```python
from build123d import *

# Parameters (mm, degrees)
F0_W     = 19.05
F0_H     = 3.429
F2_W     = 17.526
F2_H     = 2.413
F4_W     = 16.002
F4_H     = 2.413
F6_R     = 1.7399
F7_DEPTH = 8.256


with BuildPart() as f1:
    # F0 (on Front) → F1 (revolve)
    with BuildSketch(Plane.XZ):
        with Locations((9.525, 1.7145)):
            Rectangle(F0_W, F0_H)
    revolve(axis=Axis((0, 0, 1.7145), (0, 0, 1)))

    # F2 (on Front) → F3 (revolve)
    with BuildSketch(Plane.XZ):
        with Locations((8.763, 4.6355)):
            Rectangle(F2_W, F2_H)
    revolve(axis=Axis((0, 0, 4.6355), (0, 0, 1)))

    # F4 (on Front) → F5 (revolve)
    with BuildSketch(Plane.XZ):
        with Locations((8.001, 7.0485)):
            Rectangle(F4_W, F4_H)
    revolve(axis=Axis((0, 0, 7.0485), (0, 0, 1)))

    # F6 (on face) → F7 (cut, through all)
    with BuildSketch(Plane.XY.offset(8.255)):
        with Locations((8.243714, 4.308599)):
            Circle(F6_R)
    extrude(amount=-F7_DEPTH, mode=Mode.SUBTRACT)


solid = f1.part
```
Can you work these out from the model? Positions are in its coordinate system, mm. A direction names the side the tool comes from. Give positions to 0.01 mm unless a question says otherwise; leave off trailing zeros. Loops run counter-clockwise (first coordinate to the right, second up) from the corner with the lowest first, then second, coordinate; pieces in that order, holes last. Notation, with made-up numbers: M 67.25,-3.75 L 121.25,-3.75 A31 ccw 121.25,30.25 Z; hole C -38,71 d1. An arc over 180 degrees is marked long. Use one line per item in the form item = value. Start each with the question number.
(1) I'm going to push flat-ended pins straight in: P1, Ø4, axis at y = 6, z = 6, coming from the -X side; P2, Ø1.5, axis at y = 5, z = 7, coming from the +X side; P3, Ø1.5, axis at x = -1, z = 3, coming from the +Y side. Where does each tip first touch, or does it pass through?
(2) I want a section at A-A, the plane x = 0. Write out the boundary of the cut face in (y, z) (3 decimals), and give its area (3 significant figures).
(3) Please list where these lines run through material, in increasing order: line 1 (Z direction, x = -15.5, y = 6); line 2 (Y direction, x = -0.5, z = 3.25); line 3 (Y direction, x = 8.5, z = 2.25).
(4) Thinking about a two-plate mould opening in X: for faces 3 (the cylindrical face through (6.863, 3.25, 4.185)), 4 (the cylindrical face through (-3.47, -15.62, 7.07)), 5 (the flat face through (-17, -6, 3.429)), which applies, released by +X, released by -X, zero draft, split by the parting line, or undercut?
(5) On a 3-axis mill with a long thin cutter (end or side, diameter ignored), from which of +Z, -Z, +X, -X, +Y, -Y can I reach the whole of each face in a straight line? I mean faces 1 (the cylindrical face through (-15.12, -11.59, 1.74)), 2 (the flat face through (-7.7, -14.2, 5.842)). Say none if no direction works.
Worked out:
q1.P1 = -17.06
q1.P2 = 15.43
q1.P3 = 19.05
q2.outline = M -19.05,0 L 19.05,0 L 19.05,3.429 L 17.526,3.429 L 17.526,5.842 L 16.002,5.842 L 16.002,8.255 L -16.002,8.255 L -16.002,5.842 L -17.526,5.842 L -17.526,3.429 L -19.05,3.429 Z
q2.area = 292 mm²
q3.line_1 = 0 to 5.84
q3.line_2 = -19.04 to 19.04
q3.line_3 = -17.05 to 2.59, 6.03 to 17.05
q4.face_3 = undercut
q4.face_4 = split by the parting line
q4.face_5 = zero draft
q5.face_1 = +Z, -Z
q5.face_2 = +Z
